Autodesk Inventor part; units mm, degrees
ref_plane "Work Plane1" through (22.5, -3.5, -5.5) normal (0, 0, -1) x (0, 1, 0)
ref_plane "YZ Plane" through (0, 0, 0) normal (1, 0, 0) x (0, 1, 0)
ref_plane "XZ Plane" through (0, 0, 0) normal (0, 1, 0) x (-1, 0, 0)
sketch "Sketch1" plane through (0, 0, 0) normal (0, 0, 1) x (1, 0, 0)
  line L0 (-0.2, 0) -> (25.2, 0)
  line L1 (25.4, -1) -> (29.8, -1)
  line L2 (30, -0.8) -> (30, 3.8)
  line L3 (29.8, 4) -> (25.4, 4)
  line L4 (25.2, 3) -> (-0.2, 3)
  line L5 (-0.4, 4) -> (-4.8, 4)
  line L6 (-5, 3.8) -> (-5, -0.8)
  line L7 (-4.8, -1) -> (-0.4, -1)
  line L8 (25.1, -0.1) -> (-0.1, -0.1)
  line L9 (-0.1, -0.1) -> (-0.1, -1.1)
  line L10 (-0.1, -1.1) -> (-5.1, -1.1)
  line L11 (-5.1, -1.1) -> (-5.1, 4.1)
  line L12 (-5.1, 4.1) -> (-0.1, 4.1)
  line L13 (-0.1, 4.1) -> (-0.1, 3.1)
  line L14 (-0.1, 3.1) -> (25.1, 3.1)
  line L15 (25.1, 3.1) -> (25.1, 4.1)
  line L16 (25.1, 4.1) -> (30.1, 4.1)
  line L17 (30.1, 4.1) -> (30.1, -1.1)
  line L18 (30.1, -1.1) -> (25.1, -1.1)
  line L19 (25.1, -1.1) -> (25.1, -0.1)
  circle A0 centre (27.6, 1.5) radius 1.4
  circle A1 centre (-2.6, 1.5) radius 1.4
  line L20 (25.4, -1) -> (25.2, -0.8)
  line L21 (30, -0.8) -> (29.8, -1)
  line L22 (29.8, 4) -> (30, 3.8)
  line L23 (25.2, 3.8) -> (25.4, 4)
  line L24 (-0.4, 4) -> (-0.2, 3.8)
  line L25 (-5, 3.8) -> (-4.8, 4)
  line L26 (-4.8, -1) -> (-5, -0.8)
  line L27 (-0.2, -0.8) -> (-0.4, -1)
  line L28 (25.2, 3.8) -> (25.2, 3)
  line L29 (-0.2, 3) -> (-0.2, 3.8)
  line L30 (-0.2, -0.8) -> (-0.2, 0)
  line L31 (25.2, 0) -> (25.2, -0.8)
  point P0 (0, 0)
  dimension "d0" = 0.1
extrude "Extrusion1" add sketch "Sketch1" along normal blind 2 contours L30 L27 L7 L26 L6 L25 L5 L24 L29 L4 L28 L23 L3 L22 L2 L21 L1 L20 L31 L0 | L8 L9 L10 L11 L12 L13 L14 L15 L16 L17 L18 L19 | A0 | A1
sketch "Sketch2" plane through (0, 0, 2) normal (0, 0, 1) x (1, 0, 0)
  line L0 (25.1, -1.1) -> (30.1, -1.1)
  line L1 (30.1, -1.1) -> (30.1, 4.1)
  line L2 (30.1, 4.1) -> (25.1, 4.1)
  line L3 (25.1, 4.1) -> (25.1, 3.1)
  line L4 (25.1, 3.1) -> (-0.1, 3.1)
  line L5 (-0.1, 3.1) -> (-0.1, 4.1)
  line L6 (-0.1, 4.1) -> (-5.1, 4.1)
  line L7 (-5.1, 4.1) -> (-5.1, -1.1)
  line L8 (-5.1, -1.1) -> (-0.1, -1.1)
  line L9 (-0.1, -1.1) -> (-0.1, -0.1)
  line L10 (-0.1, -0.1) -> (25.1, -0.1)
  line L11 (25.1, -0.1) -> (25.1, -1.1)
  line L12 (-7.1, 6.1) -> (1.9, 6.1)
  line L13 (1.9, 6.1) -> (1.9, 5.1)
  line L14 (1.9, 5.1) -> (23.1, 5.1)
  line L15 (23.1, 5.1) -> (23.1, 6.1)
  line L16 (23.1, 6.1) -> (32.1, 6.1)
  line L17 (32.1, 6.1) -> (32.1, -3.1)
  line L18 (32.1, -3.1) -> (23.1, -3.1)
  line L19 (23.1, -3.1) -> (23.1, -2.1)
  line L20 (23.1, -2.1) -> (1.9, -2.1)
  line L21 (1.9, -2.1) -> (1.9, -3.1)
  line L22 (1.9, -3.1) -> (-7.1, -3.1)
  line L23 (-7.1, -3.1) -> (-7.1, 6.1)
  point P0 (0, 0)
  dimension "d3" = 2
ref_plane "Work Plane1" through (22.5, -3.5, -5.5) normal (0, 0, -1) x (0, 1, 0)
extrude "Extrusion2" add sketch "Sketch2" against normal up to surface (7.5 mm away)
sketch "Sketch3" plane through (1.9, -2.1, 2) normal (0, -1, 0) x (1, 0, 0)
  line L0 (6.9944, -4) -> (4.1, -4)
  arc A0 (8.2059, -3.4222) -> (6.9944, -4) centre (10.6, -10) ccw
  arc A1 (10.6, -3) -> (8.2059, -3.4222) centre (10.6, -10) ccw
  arc A2 (10.6, -3) -> (8.2059, -3.4222) centre (10.6, -10) ccw
  arc A3 (12.9941, -3.4222) -> (10.6, -3) centre (10.6, -10) ccw
  circle A4 centre (10.6, -10) radius 5.6
  arc A5 (14.2056, -4) -> (12.9941, -3.4222) centre (10.6, -10) ccw
  line L1 (17.1, -4) -> (14.2056, -4)
  line L2 (17.1, -7.4019) -> (17.1, -4)
  line L3 (4.1, -4) -> (4.1, -7.4019)
  circle A6 centre (10.6, -10) radius 5.6
  arc A7 (4.1, -7.4019) -> (3.8918, -8) centre (10.6, -10) ccw
  arc A8 (17.3082, -8) -> (17.1, -7.4019) centre (10.6, -10) ccw
  arc A9 (7.8638, -2.4825) -> (6.727, -3) centre (10.6, -10) ccw
  line L4 (6.727, -3) -> (3.1, -3)
  line L5 (3.1, -3) -> (3.1, -7.2161)
  arc A10 (3.1, -7.2161) -> (2.9335, -7.7143) centre (10.6, -10) ccw
  arc A11 (10.6, -2) -> (7.8638, -2.4825) centre (10.6, -10) ccw
  arc A12 (13.3362, -2.4825) -> (10.6, -2) centre (10.6, -10) ccw
  arc A13 (14.473, -3) -> (13.3362, -2.4825) centre (10.6, -10) ccw
  line L6 (14.473, -3) -> (18.1, -3)
  line L7 (18.1, -3) -> (18.1, -7.2161)
  arc A14 (18.2665, -7.7143) -> (18.1, -7.2161) centre (10.6, -10) ccw
  line L8 (0, -7.5) -> (21.2, -7.5)
  point P0 (-1.9, -2)
  point P1 (17.1383, -7.5)
  point P2 (18.1993, -7.5)
  point P3 (10.6, -2)
  point P4 (7.8638, -2.4825)
  point P5 (3.0007, -7.5)
  point P6 (4.0617, -7.5)
  dimension "d6" = 1
  dimension "d7" = 1
  dimension "d8" = 1
extrude "Extrusion3" cut sketch "Sketch3" against normal blind 10 contours A0 A1 A3 A5 L1 L2 A8 L8 A4 A7 L3 L0 | L0 L3 A7 L8 A10 L5 L4 A9 A11 A12 A13 L6 L7 A14 A8 L2 L1 A5 A3 A1 A0 | A4 L8 picked at (9.9261, -6.5925)
sketch "Sketch4" plane through (1.9, -2.1, 2) normal (0, -1, 0) x (1, 0, 0)
  line L0 (3.1, -7.2161) -> (3.1, -3)
  line L1 (0, -7.5) -> (3.0007, -7.5)
  line L2 (-9, -7.5) -> (0, -7.5)
  line L3 (-1.9, -6.3) -> (-1.9, -15)
  line L4 (18.1, -3) -> (18.1, -7.2161)
  arc A0 (3.1, -7.2161) -> (3.0007, -7.5) centre (10.6, -10) ccw
  arc A1 (18.1993, -7.5) -> (18.1, -7.2161) centre (10.6, -10) ccw
  line L5 (18.1993, -7.5) -> (21.2, -7.5)
  line L6 (21.2, -7.5) -> (30.2, -7.5)
  line L7 (23.1, -15) -> (23.1, -6.3)
  line L8 (3.1, -3) -> (-1.9, -7.5)
  line L9 (18.1, -3) -> (14.473, -3)
  line L10 (18.1, -3) -> (23.1, -7.5)
  point P0 (-1.9, -2)
extrude "Extrusion4" cut sketch "Sketch4" along normal mid plane 33.75
sketch "Sketch5" plane through (0, 0, 2) normal (0, 0, 1) x (1, 0, 0)
  line L0 (-3.9999, -1) -> (-4.8, -1)
  line L1 (-5, -0.8) -> (-5, 3.8)
  line L2 (-4.8, 4) -> (-3.9999, 4)
  line L3 (28.9999, 4) -> (29.8, 4)
  line L4 (30, 3.8) -> (30, -0.8)
  line L5 (29.8, -1) -> (28.9999, -1)
  line L6 (25.2, 4) -> (30, -1)
  line L7 (-0.2, 4) -> (-5, -1)
  circle A0 centre (-2.6, 1.5) radius 1.5
  circle A1 centre (27.6, 1.5) radius 1.5
  line L8 (30, 3.8) -> (29.8, 4)
  line L9 (29.8, -1) -> (30, -0.8)
  line L10 (-5, -0.8) -> (-4.8, -1)
  line L11 (-4.8, 4) -> (-5, 3.8)
  arc A2 (-3.9999, 1.5167) -> (-3.9999, 1.4833) centre (-2.6, 1.5) ccw
  line L12 (-3.9999, 1.5167) -> (-3.9999, 4)
  line L13 (-3.9999, -1) -> (-3.9999, 1.4833)
  arc A3 (28.9999, 1.4833) -> (28.9999, 1.5167) centre (27.6, 1.5) ccw
  line L14 (28.9999, 1.4833) -> (28.9999, -1)
  line L15 (28.9999, 4) -> (28.9999, 1.5167)
  point P0 (-2.6, 1.5)
  point P1 (27.6, 1.5)
  dimension "d13" = 3
  dimension "d14" = 3
extrude "Extrusion5" cut sketch "Sketch5" against normal blind 33.75 contours A0 L13 A2 L12 L7 | L7 A0 | A0 L12 A2 L13 | L15 A3 L14 A1 L6 | A1 L14 A3 L15 | L6 A1
chamfer "Chamfer1" distance 0.2 angle 45 4 edges at (25.1, 3.1, -2.75) (25.1, -0.1, -2.75) (-0.1, -0.1, -2.75) (-0.1, 3.1, -2.75)
sketch "Sketch6" plane through (16.373, 3.1, -1) normal (0, -1, 0) x (1, 0, 0)
  line L0 (8.527, 1) -> (8.527, -4.41)
  line L1 (8.527, 1) -> (-3.873, 1)
  arc A0 (0, 0) -> (-3.873, 1) centre (-3.873, -7) ccw
  line L2 (0, 0) -> (3.627, 0)
  line L3 (3.627, 0) -> (8.527, -4.41)
  line L4 (8.627, -4.5) -> (8.727, -4.5)
  line L5 (8.727, -4.5) -> (8.727, 1)
  line L6 (8.727, 1) -> (8.527, 1)
  line L7 (8.527, 1) -> (8.527, -4.41)
  line L8 (8.527, -4.41) -> (8.627, -4.5)
  line L9 (8.727, 1) -> (8.727, -4.5)
  line L10 (-16.273, -4.41) -> (-16.273, 1)
  line L11 (-16.273, -4.41) -> (-11.373, 0)
  line L12 (-11.373, 0) -> (-7.746, 0)
  arc A1 (-3.873, 1) -> (-7.746, 0) centre (-3.873, -7) ccw
  line L13 (-3.873, 1) -> (-16.273, 1)
  line L14 (-16.373, -4.5) -> (-16.273, -4.41)
  line L15 (-16.273, -4.41) -> (-16.273, 1)
  line L16 (-16.273, 1) -> (-16.473, 1)
  line L17 (-16.473, 1) -> (-16.473, -4.5)
  line L18 (-16.473, -4.5) -> (-16.373, -4.5)
  point P0 (-16.373, 1)
  point P1 (-3.873, 1)
  point P2 (-3.873, 1)
  point P3 (-3.873, 1)
  point P4 (-3.873, 1)
  point P5 (8.527, 1)
extrude "Extrusion6" cut sketch "Sketch6" against normal up to surface (1 mm away)
sketch "Sketch7" plane through (16.373, -0.1, -1) normal (0, 1, 0) x (1, 0, 0)
  line L0 (-16.273, -1) -> (-16.273, 4.41)
  line L1 (-16.273, -1) -> (-3.873, -1)
  arc A0 (-7.746, 0) -> (-3.873, -1) centre (-3.873, 7) ccw
  line L2 (-7.746, 0) -> (-11.373, 0)
  line L3 (-11.373, 0) -> (-16.273, 4.41)
  line L4 (-16.373, 4.5) -> (-16.473, 4.5)
  line L5 (-16.473, 4.5) -> (-16.473, -1)
  line L6 (-16.473, -1) -> (-16.273, -1)
  line L7 (-16.273, -1) -> (-16.273, 4.41)
  line L8 (-16.273, 4.41) -> (-16.373, 4.5)
  line L9 (8.527, 4.41) -> (8.527, -1)
  line L10 (8.527, 4.41) -> (3.627, 0)
  line L11 (3.627, 0) -> (0, 0)
  arc A1 (-3.873, -1) -> (0, 0) centre (-3.873, 7) ccw
  line L12 (-3.873, -1) -> (8.527, -1)
  line L13 (8.627, 4.5) -> (8.527, 4.41)
  line L14 (8.527, 4.41) -> (8.527, -1)
  line L15 (8.527, -1) -> (8.727, -1)
  line L16 (8.727, -1) -> (8.727, 4.5)
  line L17 (8.727, 4.5) -> (8.627, 4.5)
  point P0 (-16.373, -1)
extrude "Extrusion7" cut sketch "Sketch7" against normal up to surface (1 mm away)
sketch "Sketch8" plane through (1.9, -2.1, 2) normal (0, -1, 0) x (1, 0, 0)
  line L0 (18.1, -3) -> (21.2, -5.79)
  line L1 (21.2, 0) -> (21.2, -5.79)
  line L2 (0, 0) -> (21.2, 0)
  line L3 (0, 0) -> (0, -5.79)
  line L4 (0, -5.79) -> (3.1, -3)
  line L5 (3.1, -3) -> (6.727, -3)
  arc A0 (14.473, -3) -> (6.727, -3) centre (10.6, -10) ccw
  line L6 (14.473, -3) -> (18.1, -3)
  point P0 (-1.9, -2)
extrude "Extrusion8" add sketch "Sketch8" along normal up to surface (1 mm away)
sketch "Sketch9" plane through (1.9, 5.1, 2) normal (0, 1, 0) x (1, 0, 0)
  line L0 (21.2, 5.79) -> (18.1, 3)
  line L1 (18.1, 3) -> (14.473, 3)
  arc A0 (6.727, 3) -> (14.473, 3) centre (10.6, 10) ccw
  line L2 (6.727, 3) -> (3.1, 3)
  line L3 (3.1, 3) -> (0, 5.79)
  line L4 (0, 0) -> (0, 5.79)
  line L5 (21.2, 0) -> (0, 0)
  line L6 (21.2, 0) -> (21.2, 5.79)
  point P0 (-1.9, 2)
extrude "Extrusion9" add sketch "Sketch9" along normal up to surface (1 mm away)
sketch "Sketch10" plane through (32.1, -3.1, -5.5) normal (0, 0, -1) x (-1, 0, 0)
  line L0 (37.2, 2) -> (19.6, 2)
  line L1 (37.2, 7.2) -> (37.2, 2)
  line L2 (37.2, 7.2) -> (19.6, 7.2)
  line L3 (2, 7.2) -> (19.6, 7.2)
  line L4 (2, 2) -> (2, 7.2)
  line L5 (19.6, 2) -> (2, 2)
  circle A0 centre (34.7, 4.6) radius 1.5
  circle A1 centre (4.5, 4.6) radius 1.5
  line L6 (19.6, 7.4) -> (37.4, 7.4)
  line L7 (37.4, 7.4) -> (37.4, 1.8)
  line L8 (37.4, 1.8) -> (19.6, 1.8)
  line L9 (19.6, 1.8) -> (1.8, 1.8)
  line L10 (1.8, 1.8) -> (1.8, 7.4)
  line L11 (1.8, 7.4) -> (19.6, 7.4)
  point P0 (32.1, 3.1)
  dimension "d28" = 0.2
extrude "Extrusion10" cut sketch "Sketch10" against normal up to surface (5.5 mm away) contours L0 L5 L4 L3 L2 L1 | A0 | A1 | L6 L7 L8 L9 L10 L11
properties part number "CameraTopSlider_3DPrint"
CAD build for the part. Positions are in the model's coordinates, mm. A direction names the side the tool comes from. Round coordinates to 2 decimals unless told otherwise and drop trailing zeros. Order: outer loops, then holes, each group sorted by start corner. A loop starts at its lowest first (then second) coordinate and runs counter-clockwise, first axis right, second up. Notation, with made-up numbers: (74.25, 41.25) - (109.25, 41.25) arc R32 cw to (109.25, 79.25) - close; hole circle Ø1 at (19.5, 79). An arc over 180 degrees is marked (long way). Answer as CSV lines item,"result". Start each with the question number.
1. Pin check, flat tips, straight feed: pin 1 (0.5 mm diameter, centred on x = 18, y = 5, fed in from -Z); pin 2 (3.5 mm diameter, centred on x = -2.6, y = 1.5, fed in from -Z). Stop position of each tip, or through.
2. Drill centre lines: L1, parallel to X at y = 1.5, z = 0.95; L2, parallel to X at y = -0.25, z = -2.75; L3, parallel to Y at x = -5, z = -3. Where is each one in solid material? Low to high. Write a range as [from, to].
3. Saw through at B-B, the plane x = 27.6. Write the cut outline in (y, z), and give its area (3 significant figures).
4. Saw through at D-D, the plane x = -4.5. Write the cut outline in (y, z).
5. Saw through at C-C, the plane z = 1.5. Write the cut outline in (x, y).
6. Pull direction X, two halves, no side cores. Call faces 1 (the face through (32.1, 2, -2)), 2 (the face through (13, 1, 2)), 3 (the face through (18, -2, -1)): +X half, -X half, draft (parallel to the pull), parting line (faces both ways), or undercut.
7. Tool access for faces 4 (the face through (25, -1.3, -2)), 5 (the face through (-1.17, 1.95, 1.01)), 6 (the face through (2.535, 5.187, -3.219)): list every direction of +Z, -Z, +X, -X, +Y, -Y with a clear straight run to the whole face (end or side of a thin tool).
8. Saw through at A-A, the plane y = 1.5. Write the cut outline in (x, z), and give its area (3 significant figures).
Model answer:
1,pin 1,"stops at z = -1"
1,pin 2,"stops at z = 0"
2,L1,"x = [-7.1, -4.1], [-1.1, 26.1], [29.1, 32.1]"
2,L2,"x = [-7.1, -5.3], [30.3, 32.1]"
2,L3,"y = [-3.1, -1.3], [4.3, 6.1]"
3,outline,"(-3.1, -5.5) - (-1.3, -5.5) - (-1.3, 0) - (0, 0) - (0, 2) - (-3.1, 2) - close; (3, 0) - (4.3, 0) - (4.3, -5.5) - (6.1, -5.5) - (6.1, 2) - (3, 2) - close"
3,area,"32.2 mm²"
4,outline,"(-3.1, -5.5) - (-1.3, -5.5) - (-1.3, 0) - (4.3, 0) - (4.3, -5.5) - (6.1, -5.5) - (6.1, 2) - (-3.1, 2) - close"
5,outline,"(-7.1, -3.1) - (32.1, -3.1) - (32.1, 6.1) - (-7.1, 6.1) - close; hole circle Ø3 at (-2.6, 1.5); hole circle Ø3 at (27.6, 1.5)"
6,face 1,"+X half"
6,face 2,"draft"
6,face 3,"undercut"
7,face 4,"-Z"
7,face 5,"+Z, -Z"
7,face 6,"-Z, +Y, -Y"
8,outline,"(-7.1, -5.5) - (-5.3, -5.5) - (-5.3, 0) - (-4.1, 0) - (-4.1, 2) - (-7.1, 2) - close; (-1.1, 0) - (26.1, 0) - (26.1, 2) - (-1.1, 2) - close; (29.1, 0) - (30.3, 0) - (30.3, -5.5) - (32.1, -5.5) - (32.1, 2) - (29.1, 2) - close"
8,area,"86.2 mm²"
